Here's how the part is built. I have some questions about the finished solid (model axes, mm). Face numbers are marked on the shaded views. A direction names the side the tool comes from. Coordinates: 2 decimals unless noted, no trailing zeros. Order: outer loops, then holes, each group sorted by start corner. A loop starts at its lowest first (then second) coordinate and runs counter-clockwise, first axis right, second up. Notation, with made-up numbers: (71.5, 41.25) - (93.5, 41.25) arc R5 ccw to (93.5, 49.25) - close; hole circle Ø11 at (15.5, 43). An arc over 180 degrees is marked (long way). Answer in a Markdown table with one row per item. Add a question column.
Item 1: I want a section at A-A (y = 40). Please give me the cut outline in (x, z).
Item 2: I want a section at D-D (y = 7). Please give me the cut outline in (x, z), plus the area to 3 significant figures.
Item 3: I want a section at B-B (y = 18). Please give me the cut outline in (x, z).
Item 4: I want a section at C-C (y = 32.5). Count the separate pieces of the cut face and the enclosed holes in it, plus the area to 3 significant figures.
Item 5: Thinking about a two-plate mould opening in Y: for the marked faces 1, 2 and 3, which applies, +Y half, -Y half, draft (parallel to the pull), parting line (faces both ways), or undercut?
Item 6: If I drill on line 1 along Y through (x, z) = (-1.75, 2.5); line 2 along Y through (x, z) = (-26, 3.05); line 3 along Y through (x, z) = (-4.15, 2.5), over which ranges is the centre line in solid material (lowest first)? Write a range as from..to.
Item 7: Will these pins go through, and if not, where does the flat tip stop? pin 1 Ø2 at (y, z) = (18, 2.5) entering from +X; pin 2 Ø1.9 at (x, z) = (-0.5, 1.5) entering from +Y; pin 3 Ø1 at (y, z) = (35.5, 3.5) entering from -X.
Item 8: On a 3-axis mill with a long thin cutter (end or side, diameter ignored), from which of +Z, -Z, +X, -X, +Y, -Y can I reach the whole of each face in a straight line? I mean the marked faces 4 and 5. Say none if no direction works.
Autodesk Inventor part; units mm, degrees
ref_plane "YZ Plane" through (0, 0, 0) normal (1, 0, 0) x (0, 1, 0)
ref_plane "XZ Plane" through (0, 0, 0) normal (0, 1, 0) x (-1, 0, 0)
ref_plane "XY Plane" through (0, 0, 0) normal (0, 0, 1) x (1, 0, 0)
sketch "스케치1" plane through (0, 0, 0) normal (0, 0, 1) x (1, 0, 0)
  line L0 (0, 0) -> (0, 58)
  line L1 (0, 58) -> (-1.7157, 58)
  line L2 (-15.8579, 63.8579) -> (-17.0711, 65.0711)
  line L3 (-10, 58) -> (-8.2843, 58) construction
  line L4 (-17.0711, 65.0711) -> (-58.0833, 24.0589)
  line L5 (-58.0833, 24.0589) -> (-39.8823, 5.8579)
  line L6 (-25.7401, 0) -> (0, 0)
  arc A0 (-15.8579, 63.8579) -> (-1.7157, 58) centre (-1.7157, 78) ccw
  arc A1 (-39.8823, 5.8579) -> (-25.7401, 0) centre (-25.7401, 20) ccw
  point P0 (-34.0244, 0)
  dimension "d4" = 58
  dimension "d5" = 10
  dimension "d7" = 10
  dimension "d8" = 135
  dimension "d11" = 58
  dimension "d14" = 135
  dimension "d16" = 20
  dimension "d53" = 45
extrude "돌출1" add sketch "스케치1" along normal blind 5
sketch "스케치3" plane through (0, 0, 5) normal (0, 0, 1) x (1, 0, 0)
  line L0 (-19.4302, 48.5698) -> (-40.4104, 27.5896)
  line L1 (-17.0711, 65.0711) -> (-58.0833, 24.0589)
  line L2 (-58.0833, 24.0589) -> (-39.8823, 5.8579)
  line L3 (-15.8579, 63.8579) -> (-17.0711, 65.0711)
  line L4 (-10, 44.6636) -> (-10, 14.9932)
  line L5 (0, 58) -> (-1.7157, 58)
  line L6 (-25.7401, 0) -> (0, 0)
  line L7 (0, 0) -> (0, 58)
  line L8 (-39.7615, 24.3276) -> (-12.7654, 13.1455)
  line L9 (-11.2346, 46.5114) -> (-17.2506, 49.0033)
  arc A0 (-40.4104, 27.5896) -> (-39.7615, 24.3276) centre (-38.9962, 26.1754) ccw
  arc A1 (-12.7654, 13.1455) -> (-10, 14.9932) centre (-12, 14.9932) ccw
  arc A2 (-10, 44.6636) -> (-11.2346, 46.5114) centre (-12, 44.6636) ccw
  arc A3 (-17.2506, 49.0033) -> (-19.4302, 48.5698) centre (-18.016, 47.1556) ccw
  point P0 (-43.9411, 24.0589)
  point P1 (-36.8701, 16.9878)
  point P2 (-10, 10)
  point P3 (-20, 10)
  point P4 (-18.4853, 49.5147)
  point P5 (-42.5269, 25.4731)
  point P6 (-10, 46)
  point P7 (-10, 12)
  dimension "d17" = 10
  dimension "d20" = 10
  dimension "d23" = 10
  dimension "d24" = 10
  dimension "d52" = 2
extrude "돌출2" cut sketch "스케치3" against normal blind 6
sketch "스케치4" plane through (-58.0833, 24.0589, 0) normal (-0.7071, 0.7071, 0) x (-0.7071, -0.7071, 0)
  line L0 (-58, 0) -> (-58, 5)
  line L1 (-58, 2.5) -> (0, 2.5) construction
  line L2 (0, 0) -> (0, 5)
  circle A0 centre (-51, 2.5) radius 1.25
  circle A1 centre (-40, 2.5) radius 1.25
  circle A2 centre (-18, 2.5) radius 1.25
  circle A3 centre (-7, 2.5) radius 1.25
  point P0 (-24.0589, 0)
  dimension "d29" = 2.5
  dimension "d30" = 2.5
  dimension "d31" = 2.5
  dimension "d32" = 2.5
  dimension "d33" = 7
  dimension "d34" = 11
  dimension "d35" = 22
  dimension "d36" = 11
extrude "돌출3" cut sketch "스케치4" against normal blind 6
sketch "스케치5" plane through (0, 0, 0) normal (1, 0, 0) x (0, 0, -1)
  line L0 (0, 58) -> (-5, 58)
  line L1 (-2.5, 58) -> (-2.5, 17.6545) construction
  circle A0 centre (-2.5, 51) radius 1.25
  circle A1 centre (-2.5, 40) radius 1.25
  circle A2 centre (-2.5, 18) radius 1.25
  circle A3 centre (-2.5, 7) radius 1.25
  line L2 (0, 0) -> (-5, 0)
  dimension "d39" = 2.5
  dimension "d40" = 2.5
  dimension "d41" = 2.5
  dimension "d42" = 2.5
  dimension "d43" = 7
  dimension "d44" = 11
  dimension "d45" = 11
  dimension "d47" = 7
extrude "돌출4" cut sketch "스케치5" against normal blind 6
sketch "스케치6" plane through (0, 0, 0) normal (1, 0, 0) x (0, 0, -1)
  circle A0 centre (-2.5, 40) radius 1.25
  circle A1 centre (-2.5, 18) radius 1.25
  circle A2 centre (-2.5, 51) radius 1.25
  circle A3 centre (-2.5, 7) radius 1.25
  line L0 (0, 0) -> (0, 58)
  line L1 (0, 58) -> (-5, 58)
  line L2 (-5, 0) -> (-5, 58)
  line L3 (0, 0) -> (-5, 0)
properties part number "조인트3_박스사이드_6T" material "알루미늄 6061"
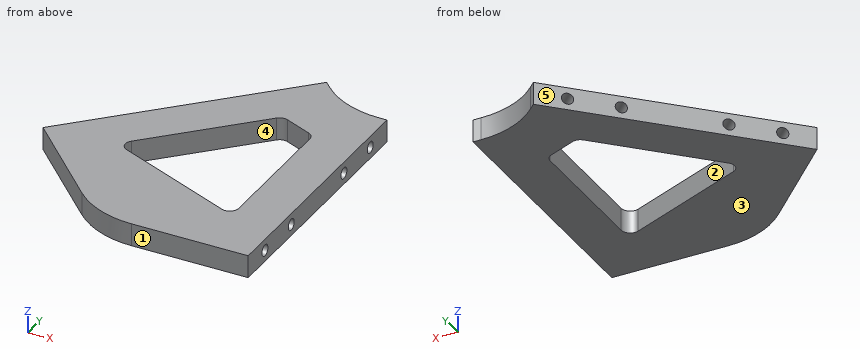
Values follow:
| question | item | result |
|---|---|---|
| 1 | outline | (-42.14, 0) - (-28, 0) - (-28, 5) - (-42.14, 5) - close; (-10, 0) - (0, 0) - (0, 1.25) - (-6, 1.25) - (-6, 3.75) - (0, 3.75) - (0, 5) - (-10, 5) - close |
| 2 | outline | (-41.02, 0) - (0, 0) - (0, 1.25) - (-6, 1.25) - (-6, 3.75) - (0, 3.75) - (0, 5) - (-41.02, 5) - close |
| 2 | area | 190 mm^2 |
| 3 | outline | (-52.02, 0) - (-24.49, 0) - (-24.49, 5) - (-52.02, 5) - close; (-10, 0) - (0, 0) - (0, 1.25) - (-6, 1.25) - (-6, 3.75) - (0, 3.75) - (0, 5) - (-10, 5) - close |
| 4 | separate pieces | 2 |
| 4 | enclosed holes | 1 |
| 4 | area | 117 mm^2 |
| 5 | face 1 | -Y half |
| 5 | face 2 | undercut |
| 5 | face 3 | draft |
| 6 | line 1 | y = 0..5.75, 8.25..16.75, 19.25..38.75, 41.25..49.75, 52.25..58 |
| 6 | line 2 | y = 0..18.63, 42..47.65, 50.13..56.14 |
| 6 | line 3 | y = 0..5.75, 8.25..16.75, 19.25..38.75, 41.25..49.75, 52.25..58.15 |
| 7 | pin 1 | stops at x = -6 |
| 7 | pin 2 | stops at y = 58 |
| 7 | pin 3 | stops at x = -47.14 |
| 8 | face 4 | +Z, -Z |
| 8 | face 5 | +Z, -Z, -X, +Y |
